Part model, mm, in its own coordinate system. Face numbers are marked on the shaded views. A direction names the side the tool comes from. Coordinates: 2 decimals unless noted, no trailing zeros. Order: outer loops, then holes, each group sorted by start corner. A loop starts at its lowest first (then second) coordinate and runs counter-clockwise, first axis right, second up. Notation, with made-up numbers: (38.5, 38) - (97.5, 38) arc R28 cw to (97.5, 70) - close; hole circle Ø6 at (-11, -18.5). An arc over 180 degrees is marked (long way). Use a Markdown table: item, result. Add a question column.
1) Tool access for the marked faces 4 and 5: list every direction of +Z, -Z, +X, -X, +Y, -Y with a clear straight run to the whole face (end or side of a thin tool).
2) Saw through at B-B on x = -207.5. List the corners of the cut face in (y, z) (3 decimals).
3) Drop a flat-ended pin along its axis: P1, Ø6, axis at x = 162.5, z = -231, coming from the +Y side (3 decimals). Give the stop position or say it passes through.
4) Saw through at C-C on z = 136. List the corners of the cut face in (x, y) (3 decimals), then the cut area to 3 significant figures.
5) Wall check: L1, parallel to Y at x = 264, z = -25; L2, parallel to Z at x = 265, y = 31; L3, parallel to Y at x = -265.9, z = -76.2. Give the ranges that are in metal, low to high. Write a range as [from, to].
6) Saw through at A-A on z = -178.5. List the corners of the cut face in (x, y) (3 decimals), then the cut area to 3 significant figures.
7) Two-plate mould, pull along X, no slides. Class the marked faces 1, 2 and 3: +X half, -X half, draft (parallel to the pull), parting line (faces both ways), or undercut.
Autodesk Inventor part; units mm, degrees
ref_plane "XZ Plane" through (0, 0, 0) normal (0, 1, 0) x (-1, 0, 0)
sketch "Sketch1" plane through (0, 0, 0) normal (0, 0, 1) x (1, 0, 0)
  line L0 (0, 0) -> (-266.7, 0)
  line L1 (-266.7, 0) -> (-266.7, 101.6)
  line L2 (-266.7, 101.6) -> (-263.525, 101.6)
  line L3 (-263.525, 101.6) -> (-263.525, 3.175)
  line L4 (0, 0) -> (0, 3.175) construction
  line L5 (0, 3.175) -> (-263.525, 3.175)
  line L6 (0, 0) -> (266.7, 0)
  line L7 (266.7, 0) -> (266.7, 101.6)
  line L8 (266.7, 101.6) -> (263.525, 101.6)
  line L9 (263.525, 101.6) -> (263.525, 3.175)
  line L10 (0, 3.175) -> (263.525, 3.175)
  dimension "d0" = 101.6
  dimension "d1" = 266.7
  dimension "d2" = 3.175
  dimension "d4" = 3.175
extrude "Extrusion1" add sketch "Sketch1" along normal mid plane 711.2
fillet "Fillet1" radius 3.175 2 edges at (-263.525, 3.175, 0) (263.525, 3.175, 0)
sketch "Sketch5" plane through (-263.525, 101.6, 355.6) normal (1, 0, 0) x (0, 0, -1)
  circle A0 centre (12.7, -34.925) radius 2.5527
  circle A1 centre (22.225, -25.4) radius 2.5527
  circle A2 centre (31.75, -15.875) radius 2.5527
  circle A3 centre (50.8, -15.875) radius 3.3782
  circle A4 centre (76.2, -15.875) radius 3.7287
  circle A5 centre (12.7, -88.9) radius 2.667
  circle A6 centre (22.225, -79.375) radius 2.667
  circle A7 centre (31.75, -69.85) radius 2.5527
  circle A8 centre (50.8, -82.55) radius 3.8164
  circle A9 centre (76.2, -88.9) radius 3.3782
  circle A10 centre (101.4806, -93.6752) radius 3.3782
  circle A11 centre (212.631, -93.6752) radius 3.3782
  circle A12 centre (228.6, -88.9) radius 3.7287
  circle A13 centre (279.4, -86.36) radius 3.8164
  circle A14 centre (228.6, -15.875) radius 3.3782
  circle A15 centre (254, -15.875) radius 3.7287
  circle A16 centre (279.4, -15.875) radius 3.3782
  circle A17 centre (304.8, -15.875) radius 3.3782
  circle A18 centre (330.2, -15.875) radius 3.7287
  circle A19 centre (355.6, -15.875) radius 3.3782
  circle A20 centre (381, -15.875) radius 3.3782
  circle A21 centre (431.8, -15.875) radius 3.7287
  circle A22 centre (454.025, -19.05) radius 3.8164
  circle A23 centre (508, -82.55) radius 3.8164
  circle A24 centre (457.2, -88.9) radius 3.3782
  circle A25 centre (431.8, -88.9) radius 3.7287
  circle A26 centre (475.0995, -43.8435) radius 3.3782
  circle A27 centre (412.75, -42.8625) radius 2.5527
  circle A28 centre (403.225, -52.3875) radius 2.667
  circle A29 centre (393.7, -61.9125) radius 2.5527
  circle A30 centre (381, -88.9) radius 3.3782
  circle A31 centre (355.6, -88.9) radius 3.3782
  circle A32 centre (330.2, -88.9) radius 3.7287
  circle A33 centre (304.8, -88.9) radius 3.3782
  circle A34 centre (492.125, -82.55) radius 4.826
  circle A35 centre (508, -82.55) radius 5.2255
  point P0 (355.6, -101.6)
extrude "Extrusion5" cut sketch "Sketch5" along normal through all both and the other way through all
sketch "Sketch12" plane through (-263.525, 19.05, -152.4) normal (1, 0, 0) x (0, 0, -1)
  circle A0 centre (0, 0) radius 4.2111
  point P0 (-152.4, -19.05)
extrude "Extrusion10" cut sketch "Sketch12" along normal through all both and the other way through all
sketch "Sketch25" plane through (-266.7, 0, 355.6) normal (-1, 0, 0) x (0, 0, 1)
  line L0 (-711.2, 3.175) -> (0, 3.175)
  line L1 (0, 101.6) -> (-711.2, 101.6)
  line L2 (-241.3, 3.175) -> (-88.9, 3.175)
  line L3 (-88.9, 3.175) -> (-88.9, 63.5)
  line L4 (-88.9, 101.6) -> (-241.3, 101.6)
  line L5 (-241.3, 101.6) -> (-241.3, 3.175)
  line L6 (0, 101.6) -> (0, 0)
  line L7 (0, 101.6) -> (-88.9, 101.6)
  line L8 (-88.9, 63.5) -> (0, 63.5)
  line L9 (0, 63.5) -> (0, 101.6)
  point P0 (-355.6, 0)
  dimension "d81" = 88.9
  dimension "d82" = 241.3
  dimension "d83" = 38.1
extrude "Extrusion22" cut sketch "Sketch25" against normal through all contours L5 L1 L6 L8 L3 L0
equation "\"BendRadius\" = Thickness"
equation "\"BendReliefWidth\" = Thickness"
equation "\"BendReliefDepth\" = 0.5 * Thickness"
equation "\"CornerReliefSize\" = 4 * Thickness"
equation "\"MinimumRemnant\" = 2 * Thickness"
equation "\"TransitionRadius\" = BendRadius"
equation "\"JacobiRadiusSize\" = BendRadius"
equation "\"GapSize\" = Thickness"
properties part number "SheetBottomFloor" material "Aluminum 6061"
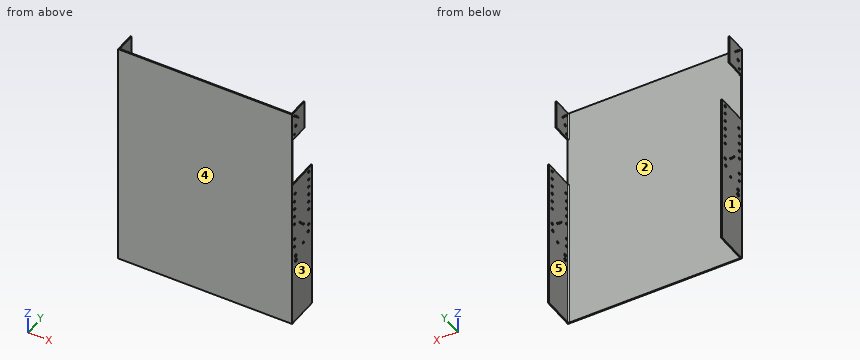
Results are:
| question | item | result |
|---|---|---|
| 1 | face 4 | +Z, -Z, +X, -X, -Y |
| 1 | face 5 | +Z, -Z, +Y |
| 2 | outline | (0, -355.6) - (3.175, -355.6) - (3.175, 355.6) - (0, 355.6) - close |
| 3 | P1 | y = 3.175 |
| 4 | outline | (-266.7, 0) - (266.7, 0) - (266.7, 3.175) - (-266.7, 3.175) - close |
| 4 | area | 1,690 mm2 |
| 5 | L1 | [0, 9.35], [16.05, 82.37], [89.08, 101.6] |
| 5 | L2 | [-355.6, 114.3], [266.7, 321.41], [326.29, 355.6] |
| 5 | L3 | [0, 8.97], [16.43, 82], [89.45, 101.6] |
| 6 | outline | (-266.7, 0) - (266.7, 0) - (266.7, 101.6) - (263.525, 101.6) - (263.525, 6.35) arc R3.175 cw to (260.35, 3.175) - (-260.35, 3.175) arc R3.175 cw to (-263.525, 6.35) - (-263.525, 101.6) - (-266.7, 101.6) - close |
| 6 | area | 2,320 mm2 |
| 7 | face 1 | -X half |
| 7 | face 2 | undercut |
| 7 | face 3 | +X half |
